For this review, take the finished solid that the model builds, in its own axes (mm). A direction names the side the tool comes from. Coordinates: 2 decimals unless noted, no trailing zeros. Write each loop counter-clockwise with the first axis right and the second up, starting at its lowest first coordinate (ties: lowest second). Pieces come first, ordered by that corner, then holes. Notation, with made-up numbers: M 86.25,24 L 108.25,24 A22 cw 108.25,37 Z; hole C 83.5,-19 d4. An arc over 180 degrees is marked long. Return JSON: item names as keys, results as strings.
```python
from build123d import *

# Parameters (mm, degrees)
BOSS_EXTRU_1_DEPTH      = 15
ENL_V_START             = -12
ESQUISSE4_R             = 1.5
ENL_V_MAT_EXTRU_4_DEPTH = 8
BOSS_EXTRU_2_DEPTH      = 20
CONG_5_R                = 1.8
ENL_V_START_2           = 15
ENL_V_MAT_EXTRU_5_DEPTH = 5
ESQUISSE7_R             = 1.5
ESQUISSE7_W             = 1.9
ESQUISSE7_H             = 0.1
ENL_V_MAT_EXTRU_6_DEPTH = 3
CONG_6_R                = 3
ESQUISSE8_R             = 0.75
ENL_V_MAT_EXTRU_7_DEPTH = 33.478642206


with BuildPart() as part:
    # Esquisse2 → Boss.-Extru.1 (new body)
    with BuildSketch(Plane(origin=(0, 0, 0), x_dir=(1, 0, 0), z_dir=(0, 1, 0))):
        Polygon((15, 12), (-15, 12), (-17.892304845, 6.990381057), (-2.892304845, -18.990381057), (2.892304845, -18.990381057), (17.892304845, 6.990381057), align=None)
        with BuildLine():
            add(Edge.make_bspline(
                [(-6.497795886, -0.435512169), (-6.562859024, 2.121494549), (-5.630578833, 3.64576447), (-3.901472034, 5.989881763), (-2.755958224, 6.442764065), (-0.876549045, 6.455616827), (1.132269087, 6.456305133), (2.764590803, 6.437211677), (3.915516646, 5.93683695), (5.68604085, 3.725822495), (6.557016299, 1.367317423), (6.496525421, -0.463293017), (6.514589536, -1.131908623), (6.247808359, -3.89361975), (4.327528544, -6.639389687), (0.544504956, -7.076982092), (-0.422677641, -7.064388331), (-3.088953313, -6.935277121), (-6.120558637, -4.860976426), (-6.514763181, -1.229822437), (-6.49155978, -0.658277257), (-6.497231202, -0.457704464), (-6.497795886, -0.435512169)],
                knots=[0, 0, 0, 0, 0.112371839, 0.130275732, 0.173620802, 0.187168536, 0.252205347, 0.266940035, 0.319780728, 0.343419676, 0.479690568, 0.498676785, 0.51429563, 0.54296722, 0.756721096, 0.785787005, 0.804560399, 0.825241089, 0.971913217, 0.99122251, 0.999024723, 1, 1, 1, 1], degree=3))
        make_face(mode=Mode.SUBTRACT)
    extrude(amount=BOSS_EXTRU_1_DEPTH)

    # Esquisse4 → Enlèv. mat.-Extru.4 (cut)
    with BuildSketch(Plane.XY.offset(ENL_V_START)):
        with Locations((-11, 11)):
            Circle(ESQUISSE4_R)
        with Locations((11, 11)):
            Circle(ESQUISSE4_R)
        with Locations((11, 3)):
            Circle(ESQUISSE4_R)
        with Locations((-11, 3)):
            Circle(ESQUISSE4_R)
    extrude(amount=ENL_V_MAT_EXTRU_4_DEPTH, mode=Mode.SUBTRACT)

    # Esquisse5 → Boss.-Extru.2 (add)
    with BuildSketch(Plane(origin=(0, 0, 0), x_dir=(1, 0, 0), z_dir=(0, 1, 0))):
        with BuildLine():
            Line((13.220508076, -17.101408311), (15.370508076, -13.377499075))
            ThreePointArc((15.370508076, -13.377499075), (15.510368667, -12.315152412), (14.85807251, -11.465063509))
            Line((14.85807251, -11.465063509), (14.68486743, -11.365063509))
            ThreePointArc((14.68486743, -11.365063509), (14.032571273, -10.514974607), (14.172431864, -9.452627944))
            Line((14.172431864, -9.452627944), (15.272431864, -7.547372056))
            ThreePointArc((15.272431864, -7.547372056), (16.122520766, -6.895075899), (17.18486743, -7.034936491))
            Line((17.18486743, -7.034936491), (17.35807251, -7.134936491))
            ThreePointArc((17.35807251, -7.134936491), (18.420419174, -7.274797082), (19.270508076, -6.622500925))
            Line((19.270508076, -6.622500925), (21.420508076, -2.898591689))
            ThreePointArc((21.420508076, -2.898591689), (21.600328836, -1.532717408), (20.761662349, -0.439745962))
            Line((20.761662349, -0.439745962), (20.415252187, -0.239745962))
            ThreePointArc((20.415252187, -0.239745962), (19.049377906, -0.059925202), (17.956406461, -0.898591689))
            Line((17.956406461, -0.898591689), (17.756406461, -1.24500185))
            ThreePointArc((17.756406461, -1.24500185), (16.663435015, -2.083668338), (15.297560734, -1.903847577))
            Line((15.297560734, -1.903847577), (13.392304845, -0.803847577))
            Line((13.392304845, -0.803847577), (7.392304845, -11.196152423))
            Line((7.392304845, -11.196152423), (9.297560734, -12.296152423))
            ThreePointArc((9.297560734, -12.296152423), (10.136227221, -13.389123868), (9.956406461, -14.75499815))
            Line((9.956406461, -14.75499815), (9.756406461, -15.101408311))
            ThreePointArc((9.756406461, -15.101408311), (9.5765857, -16.467282592), (10.415252187, -17.560254038))
            Line((10.415252187, -17.560254038), (10.761662349, -17.760254038))
            ThreePointArc((10.761662349, -17.760254038), (12.12753663, -17.940074798), (13.220508076, -17.101408311))
        make_face()
        with BuildLine():
            Line((-19.270508076, -6.622500925), (-21.420508076, -2.898591689))
            ThreePointArc((-21.420508076, -2.898591689), (-21.600328836, -1.532717408), (-20.761662349, -0.439745962))
            Line((-20.761662349, -0.439745962), (-20.415252187, -0.239745962))
            ThreePointArc((-20.415252187, -0.239745962), (-19.049377906, -0.059925202), (-17.956406461, -0.898591689))
            Line((-17.956406461, -0.898591689), (-17.756406461, -1.24500185))
            ThreePointArc((-17.756406461, -1.24500185), (-16.663435015, -2.083668338), (-15.297560734, -1.903847577))
            Line((-15.297560734, -1.903847577), (-13.392304845, -0.803847577))
            Line((-13.392304845, -0.803847577), (-7.392304845, -11.196152423))
            Line((-7.392304845, -11.196152423), (-9.297560734, -12.296152423))
            ThreePointArc((-9.297560734, -12.296152423), (-10.136227221, -13.389123868), (-9.956406461, -14.75499815))
            Line((-9.956406461, -14.75499815), (-9.756406461, -15.101408311))
            ThreePointArc((-9.756406461, -15.101408311), (-9.5765857, -16.467282592), (-10.415252187, -17.560254038))
            Line((-10.415252187, -17.560254038), (-10.761662349, -17.760254038))
            ThreePointArc((-10.761662349, -17.760254038), (-12.12753663, -17.940074798), (-13.220508076, -17.101408311))
            Line((-13.220508076, -17.101408311), (-15.370508076, -13.377499075))
            ThreePointArc((-15.370508076, -13.377499075), (-15.510368667, -12.315152412), (-14.85807251, -11.465063509))
            Line((-14.85807251, -11.465063509), (-14.68486743, -11.365063509))
            ThreePointArc((-14.68486743, -11.365063509), (-14.032571273, -10.514974607), (-14.172431864, -9.452627944))
            Line((-14.172431864, -9.452627944), (-15.272431864, -7.547372056))
            ThreePointArc((-15.272431864, -7.547372056), (-16.122520766, -6.895075899), (-17.18486743, -7.034936491))
            Line((-17.18486743, -7.034936491), (-17.35807251, -7.134936491))
            ThreePointArc((-17.35807251, -7.134936491), (-18.420419174, -7.274797082), (-19.270508076, -6.622500925))
        make_face()
    extrude(amount=BOSS_EXTRU_2_DEPTH)

    # Congé5
    cong_5_edges = [part.edges().sort_by_distance(p)[0] for p in [
        (7.392304845, 7.5, 11.196152423),
        (13.392304845, 7.5, 0.803847577),
        (-13.392304845, 7.5, 0.803847577),
        (-7.392304845, 7.5, 11.196152423),
    ]]
    fillet(cong_5_edges, radius=CONG_5_R)

    # Esquisse6 → Enlèv. mat.-Extru.5 (cut)
    with BuildSketch(Plane(origin=(0, 0, 0), x_dir=(1, 0, 0), z_dir=(0, 1, 0)).offset(ENL_V_START_2)):
        Polygon((-13.392304845, -0.803847577), (-7.392304845, -11.196152423), (-7.478907386, -11.246152423), (-13.478907386, -0.853847577), align=None)
        Polygon((7.392304845, -11.196152423), (13.392304845, -0.803847577), (13.478907386, -0.853847577), (7.478907386, -11.246152423), align=None)
    extrude(amount=ENL_V_MAT_EXTRU_5_DEPTH, mode=Mode.SUBTRACT)

    # Esquisse7 → Enlèv. mat.-Extru.6 (cut)
    # profile 1 of 3: a face of its own
    with BuildSketch(Plane(origin=(0, 0, -12), x_dir=(-1, 0, 0), z_dir=(0, 0, -1))):
        Polygon((15, 0), (0.85, 0), (-0.85, 0), (-15, 0), (-15, 14.1), (-15.1, 14.1), (-15.1, -0.1), (15.1, -0.1), (15.1, 14.1), (15, 14.1), align=None)
    # profile 2 of 3: a face of its own
    with BuildSketch(Plane(origin=(0, 0, -12), x_dir=(-1, 0, 0), z_dir=(0, 0, -1))):
        Polygon((-0.85, 0), (0.85, 0), (15, 0), (15, 14.1), (0.95, 14.1), (0.95, 15), (-0.95, 15), (-0.95, 14.1), (-15, 14.1), (-15, 0), align=None)
        with Locations((-11, 3)):
            Circle(ESQUISSE7_R, mode=Mode.SUBTRACT)
        with Locations((11, 3)):
            Circle(ESQUISSE7_R, mode=Mode.SUBTRACT)
        with Locations((-11, 11)):
            Circle(ESQUISSE7_R, mode=Mode.SUBTRACT)
        with Locations((11, 11)):
            Circle(ESQUISSE7_R, mode=Mode.SUBTRACT)
    # profile 3 of 3: a face of its own
    with BuildSketch(Plane(origin=(0, 0, -12), x_dir=(-1, 0, 0), z_dir=(0, 0, -1))):
        with Locations((0, 15.05)):
            Rectangle(ESQUISSE7_W, ESQUISSE7_H)
    extrude(amount=-ENL_V_MAT_EXTRU_6_DEPTH, mode=Mode.SUBTRACT)

    # Congé6
    cong_6_edges = [part.edges().sort_by_distance(p)[0] for p in [
        (-15.1, 14.1, -10.41339746),
        (15.1, 14.1, -10.41339746),
    ]]
    fillet(cong_6_edges, radius=CONG_6_R)

    # Esquisse8 → Enlèv. mat.-Extru.7 (cut, through all)
    with BuildSketch(Plane(origin=(0, 15, 0), x_dir=(1, 0, 0), z_dir=(0, 1, 0))):
        with Locations((-1.7, -6.924152718)):
            Circle(ESQUISSE8_R)
        with Locations((1.7, -6.924152718)):
            Circle(ESQUISSE8_R)
    extrude(amount=-ENL_V_MAT_EXTRU_7_DEPTH, mode=Mode.SUBTRACT)


solid = part.part
```
1. Draft analysis for pull direction X (two halves, no side actions). For faces 1 (the face through (20.33, 9.86, 4.79)), 2 (the face through (-14.037, 9.86, 10.53)), 3 (the face through (1.84, 7.6, 7.66)), state which applies: +X half, -X half, draft (parallel to the pull), parting line (faces both ways), or undercut.
Checks:
{"face 1": "+X half", "face 2": "-X half", "face 3": "undercut"}
2. For faces 4 (the face through (-14.715, 9.86, 8.513)), 5 (the face through (10.52, 17.46, 5.98)), 6 (the face through (14.118, 7.605, 0.63)), 7 (the face through (-12.5, 11.07, -6.54)), 8 (the face through (-8.78, 16.527, 11.997)), list the 3-axis set-ups (+Z, -Z, +X, -X, +Y, -Y) from which the entire face can be reached by the end or side of a thin tool; tool diameter is ignored.
Checks:
{"face 4": "-X, +Y, -Y", "face 5": "-Z, +Y", "face 6": "+Y, -Y", "face 7": "-Z", "face 8": "+Z, +Y"}
3. We need section B-B (x = 7). State the section outline as (y, z) points.
Checks:
{"outline": "M 0,-9 L 14.1,-9 L 14.1,-12 L 15,-12 L 15,12.19 L 0,12.19 Z"}
4. Clearance check with flat-ended pins moving along their axes: pin 1 Ø3.5 at (x, y) = (11, 11) entering from +Z; pin 2 Ø2.5 at (x, y) = (11, 3) entering from -Z; pin 3 Ø4 at (x, y) = (-11, 11) entering from -Z. State where each tip first meets the part, or that it passes through.
Checks:
{"pin 1": "z = 18", "pin 2": "z = -4", "pin 3": "z = -9"}
5. We need section A-A (z = -8). State the section outline as (x, y) points.
Checks:
{"outline": "M -17.31,0 L 17.31,0 L 17.31,15 L -17.31,15 Z; hole C -11,3 d3; hole C -11,11 d3; hole C 11,3 d3; hole C 11,11 d3"}
6. Wall thickness on L1, parallel to Y at x = -11, z = -6.45; L2, parallel to X at y = 6.25, z = 1; L3, parallel to Y at x = 6.5, z = -3: over which ranges is each line inside the solid? List them lowest first. Write a range as from..to.
Checks:
{"L1": "0..1.5, 4.5..9.5, 12.5..15", "L2": "-21.36..-17.9, -14.27..-6.5, 6.5..14.27, 17.9..21.36", "L3": "0..15"}
